Check sheet for the modelled part. Datum: model origin and axes. Units: mm. Round coordinates to 2 decimals unless told otherwise and drop trailing zeros. Answer in a Markdown table with one row per item. Add a question column.
(1) Mould release check, pull along X, two halves, no side actions. Record for faces 1 (the cylindrical face through (-51.293, 0.85, 51.34)), 2 (the flat face through (-1, 0, -1)): +X half, -X half, draft (parallel to the pull), parting line (faces both ways), or undercut.
(2) Thickness scan on line 1 along X through (y, z) = (0.85, 52); line 2 along X through (y, z) = (1.3, 50); line 3 along Z through (x, y) = (-54, 0.3). Record the ranges inside material, lowest first.
(3) Gauge pin test, flat ends, axial feed: pin 1 (6.5 mm diameter, centred on x = 56.72, z = 51.08, fed in from +Y); pin 2 (3 mm diameter, centred on x = 57.27, z = -51.42, fed in from -Y). Record the tip position at first contact, or that the pin passes through.
from build123d import *

# Parameters (mm, degrees)
SKETCH1_W           = 135
SKETCH1_H           = 114.3
BOSS_EXTRUDE1_DEPTH = 1.724
SKETCH3_W           = 135
SKETCH3_H           = 3
CUT_EXTRUDE2_DEPTH  = 0.0001
SKETCH4_R           = 2
CUT_EXTRUDE3_DEPTH  = 89.460978267


with BuildPart() as part:
    # Sketch1 → Boss-Extrude1 (new body)
    with BuildSketch(Plane(origin=(0, 0, 0), x_dir=(1, 0, 0), z_dir=(0, 1, 0))):
        Rectangle(SKETCH1_W, SKETCH1_H)
    extrude(amount=BOSS_EXTRUDE1_DEPTH)

    # Sketch3 → Cut-Extrude2 (cut)
    with BuildSketch(Plane(origin=(0, 1.724, 0), x_dir=(1, 0, 0), z_dir=(0, 1, 0))):
        with Locations((0, 55.65)):
            Rectangle(SKETCH3_W, SKETCH3_H)
        with Locations((0, -55.65)):
            Rectangle(SKETCH3_W, SKETCH3_H)
    extrude(amount=-CUT_EXTRUDE2_DEPTH, mode=Mode.SUBTRACT)

    # Sketch4 → Cut-Extrude3 (cut, through all)
    with BuildSketch(Plane.XZ):
        with Locations(Location((-53.275487911, 51.079761641, 0), (0, 0, 270))):
            Circle(SKETCH4_R)
        with Locations(Location((56.724512089, 51.079761641, 0), (0, 0, 270))):
            Circle(SKETCH4_R)
        with Locations(Location((57.272512089, -51.420238359, 0), (0, 0, 270))):
            Circle(SKETCH4_R)
        with Locations(Location((-62.927487911, -27.420238359, 0), (0, 0, 270))):
            Circle(SKETCH4_R)
    extrude(amount=-CUT_EXTRUDE3_DEPTH, mode=Mode.SUBTRACT)


solid = part.part
Answers:
| question | item | result |
|---|---|---|
| 1 | face 1 | undercut |
| 1 | face 2 | draft |
| 2 | line 1 | x = -67.5 to -55.05, -51.5 to 54.95, 58.5 to 67.5 |
| 2 | line 2 | x = -67.5 to -54.96, -51.59 to 55.04, 58.41 to 67.5 |
| 2 | line 3 | z = -57.15 to 49.22, 52.94 to 57.15 |
| 3 | pin 1 | stops at y = 1.72 |
| 3 | pin 2 | passes through |
